The model under review builds one solid part; all positions refer to its coordinate system, in mm. A direction names the side the tool comes from. Coordinates: 2 decimals unless noted, no trailing zeros. Write each loop counter-clockwise with the first axis right and the second up, starting at its lowest first coordinate (ties: lowest second). Pieces come first, ordered by that corner, then holes. Notation, with made-up numbers: (-5, 85.5) -> (3, 85.5) arc R18 ccw to (3, 101.5) -> close; hole circle Ø6 at (1.25, -18.5). An arc over 180 degrees is marked (long way). Write each question's results on one line, items separated by ' | '.
```python
from build123d import *

# Parameters (mm, degrees)
BOSS_EXTRUDE1_DEPTH = 20
SKETCH2_R           = 3
CUT_EXTRUDE5_DEPTH  = 117
CUT_EXTRUDE6_START  = -10
SKETCH5_R           = 7.5
CUT_EXTRUDE6_DEPTH  = 107
SKETCH6_R           = 3
CUT_EXTRUDE7_DEPTH  = 117
CUT_EXTRUDE8_START  = -10
SKETCH7_R           = 7.5
CUT_EXTRUDE8_DEPTH  = 107


with BuildPart() as part:
    # Sketch1 → Boss-Extrude1 (new body)
    with BuildSketch(Plane(origin=(0, 0, 0), x_dir=(0, 0, -1), z_dir=(1, 0, 0))):
        with BuildLine():
            Line((0.554855898, 101.68431358), (114.554855898, 45.013454735))
            ThreePointArc((114.554855898, 45.013454735), (115.526714295, 45.058871302), (116, 45.908913684))
            Line((116, 45.908913684), (116, 66.010337689))
            ThreePointArc((116, 66.010337689), (115.850042382, 66.537051984), (115.445144102, 66.905796637))
            Line((115.445144102, 66.905796637), (1.445144102, 123.576655482))
            ThreePointArc((1.445144102, 123.576655482), (0.473285705, 123.531238916), (0, 122.681196534))
            Line((0, 122.681196534), (0, 102.579772529))
            ThreePointArc((0, 102.579772529), (0.149957618, 102.053058233), (0.554855898, 101.68431358))
        make_face()
    extrude(amount=BOSS_EXTRUDE1_DEPTH)

    # Sketch2 → Cut-Extrude5 (cut, through all)
    with BuildSketch(Plane.XY):
        with Locations((10, 112.630484531)):
            Circle(SKETCH2_R)
    extrude(amount=-CUT_EXTRUDE5_DEPTH, mode=Mode.SUBTRACT)

    # Sketch5 → Cut-Extrude6 (cut, through all)
    with BuildSketch(Plane.XY.offset(CUT_EXTRUDE6_START)):
        with Locations((10, 112.630484531)):
            Circle(SKETCH5_R)
    extrude(amount=-CUT_EXTRUDE6_DEPTH, mode=Mode.SUBTRACT)

    # Sketch6 → Cut-Extrude7 (cut, through all)
    with BuildSketch(Plane(origin=(0, 0, -116), x_dir=(-1, 0, 0), z_dir=(0, 0, -1))):
        with Locations((-10, 55.959625686)):
            Circle(SKETCH6_R)
    extrude(amount=-CUT_EXTRUDE7_DEPTH, mode=Mode.SUBTRACT)

    # Sketch7 → Cut-Extrude8 (cut, through all)
    with BuildSketch(Plane(origin=(0, 0, -116), x_dir=(-1, 0, 0), z_dir=(0, 0, -1)).offset(CUT_EXTRUDE8_START)):
        with Locations((-10, 55.959625686)):
            Circle(SKETCH7_R)
    extrude(amount=-CUT_EXTRUDE8_DEPTH, mode=Mode.SUBTRACT)


solid = part.part
```
Q1. Add section C-C (y = 62). Write out the cut boundary in (x, z), plus the area to 3 significant figures.
Solution:
outline: (0, -116) -> (20, -116) -> (20, -80.38) -> (14.45, -80.38) -> (14.45, -106) -> (5.55, -106) -> (5.55, -80.38) -> (0, -80.38) -> close | area: 485 mm²
Q2. For line 1 (X direction, y = 110, z = -12.5); line 2 (Z direction, x = 4.5, y = 58); line 3 (Y direction, x = 10, z = -112.5), list the stretches that pass through material, from the lowest coordinate up. Write a range as from..to.
Solution:
line 1: 0..2.98, 17.02..20 | line 2: -116..-106 | line 3: 46.03..52.96, 58.96..68.37
Q3. Add section B-B (z = -81). Write out the cut boundary in (x, y).
Solution:
outline: (0, 61.69) -> (5.17, 61.69) arc R7.5 cw to (14.83, 61.69) -> (20, 61.69) -> (20, 84.03) -> (0, 84.03) -> close
Q4. Clearance check with flat-ended pins moving along their axes: P1, Ø3, axis at x = 6, z = -77.5, coming from the +Y side; P2, Ø12, axis at x = 3, z = -78, coming from the +Y side; P3, Ø3, axis at x = 12, z = -39.5, coming from the +Y side. State where each tip first meets the part, or that it passes through.
Solution:
P1: y = 86.51 | P2: y = 88.5 | P3: y = 105.4
Q5. Draft analysis for pull direction Y (two halves, no side actions). For faces 1 (the flat face through (0, 87, -58)), 2 (the flat face through (9.86, 94.845, -59.243)), 3 (the cylindrical face through (9.719, 105.136, -20.926)), state which applies: pulls with the +Y half, pulls with the -Y half, needs draft (parallel to the pull), parting line crosses it, or undercut.
Solution:
face 1: needs draft | face 2: pulls with the +Y half | face 3: undercut
Q6. Add section A-A (x = 10). Write out the cut boundary in (y, z), plus the area to 3 significant figures.
Solution:
outline: (45.01, -114.55) arc R1 ccw to (45.91, -116) -> (52.96, -116) -> (52.96, -106) -> (49.27, -106) -> close; (58.96, -116) -> (66.01, -116) arc R1 ccw to (66.91, -115.45) -> (105.13, -38.55) -> (105.13, -10) -> (109.63, -10) -> (109.63, 0) -> (102.58, 0) arc R1 ccw to (101.68, -0.55) -> (63.46, -77.45) -> (63.46, -106) -> (58.96, -106) -> close; (115.63, -10) -> (119.32, -10) -> (123.58, -1.45) arc R1 ccw to (122.68, 0) -> (115.63, 0) -> close | area: 2,060 mm²
Q7. Add section D-D (x = 3.75). Write out the cut boundary in (y, z).
Solution:
outline: (45.01, -114.55) arc R1 ccw to (45.91, -116) -> (66.01, -116) arc R1 ccw to (66.91, -115.45) -> (108.48, -31.8) -> (108.48, -10) -> (116.78, -10) -> (116.78, -15.12) -> (123.58, -1.45) arc R1 ccw to (122.68, 0) -> (102.58, 0) arc R1 ccw to (101.68, -0.55) -> (60.11, -84.2) -> (60.11, -106) -> (51.81, -106) -> (51.81, -100.88) -> close
Q8. Machinability: for faces 4 (the cylindrical face through (9.719, 63.454, -94.867)), 5 (the cylindrical face through (9.35, 109.7, -4.93)), 6 (the flat face through (10, 109, -10)), which of the approach directions +Z, -Z, +X, -X, +Y, -Y give a long, thin tool a straight path to every point of the face, cutting with its end or side? Answer none if there is none.
Solution:
face 4: +Z | face 5: +Z, -Z | face 6: -Z
